Geometry check sheet. Reference: the model listing, model coordinates, mm. A direction names the side the tool comes from. Round coordinates to 2 decimals unless told otherwise and drop trailing zeros. Order: outer loops, then holes, each group sorted by start corner. A loop starts at its lowest first (then second) coordinate and runs counter-clockwise, first axis right, second up.
```python
from build123d import *

# Parameters (mm, degrees)
EXTRUDE_1_DEPTH     = 70
SKETCH_2_R          = 1.65
CUT_EXTRUDE_1_DEPTH = 25.69615506
FILLET_1_R          = 3
SKETCH_6_R          = 2.65
CUT_EXTRUDE_4_DEPTH = 31.641777725
EXTRUDE_2_DEPTH     = 3
CUT_EXTRUDE_5_DEPTH = 31.641777725


with BuildPart() as part:
    # 草图1 → 凸台-拉伸1 (new body)
    with BuildSketch(Plane(origin=(0, 0, 0), x_dir=(0, 0, -1), z_dir=(1, 0, 0))):
        Polygon((0, 0), (90, 0), (64.288495613, -30.641777725), (60.458273397, -27.427839676), (79.277465397, -5), (0, -5), align=None)
    extrude(amount=EXTRUDE_1_DEPTH)

    # 草图2 → 切除-拉伸1 (cut, through all)
    with BuildSketch(Plane(origin=(0, -41.102410837, -48.983945779), x_dir=(1, 0, 0), z_dir=(0, 0.64278761, 0.766044443))):
        with Locations((12.5, 27.850884872)):
            Circle(SKETCH_2_R)
        with Locations((57.5, 27.850884872)):
            Circle(SKETCH_2_R)
    extrude(amount=-CUT_EXTRUDE_1_DEPTH, mode=Mode.SUBTRACT)

    # 圆角1
    fillet_1_edges = [part.edges().sort_by_distance(p)[0] for p in [
        (35, 0, -90),
        (35, -5, -79.277465397),
    ]]
    fillet(fillet_1_edges, radius=FILLET_1_R)

    # 草图6 → 切除-拉伸4 (cut, through all)
    with BuildSketch(Plane(origin=(0, 0, 0), x_dir=(1, 0, 0), z_dir=(0, 1, 0))):
        with Locations((48.75, 5)):
            Circle(SKETCH_6_R)
    extrude(amount=-CUT_EXTRUDE_4_DEPTH, mode=Mode.SUBTRACT)

    # 草图7 → 凸台-拉伸2 (add)
    with BuildSketch(Plane.ZY):
        with BuildLine():
            Line((-60.458273397, -27.427839676), (-15, -5))
            Line((-15, -5), (0, -5))
            Line((0, -5), (0, 0))
            Line((0, 0), (-83.566479238, 0))
            ThreePointArc((-83.566479238, 0), (-86.2854026, -1.732145215), (-85.864612568, -4.928362829))
            Line((-85.864612568, -4.928362829), (-64.288495613, -30.641777725))
            Line((-64.288495613, -30.641777725), (-60.458273397, -27.427839676))
        make_face()
    extrude_2 = extrude(amount=EXTRUDE_2_DEPTH)

    # 镜向1: 凸台-拉伸2 across plane
    add(extrude_2.mirror(Plane.ZY.offset(-35)))

    # 草图8 → 切除-拉伸5 (cut, through all)
    with BuildSketch(Plane(origin=(0, 0, 0), x_dir=(1, 0, 0), z_dir=(0, 1, 0))):
        with BuildLine():
            Line((16.25, 10.15), (26.25, 10.15))
            ThreePointArc((26.25, 10.15), (28.9, 7.5), (26.25, 4.85))
            Line((26.25, 4.85), (16.25, 4.85))
            ThreePointArc((16.25, 4.85), (13.6, 7.5), (16.25, 10.15))
        make_face()
    extrude(amount=-CUT_EXTRUDE_5_DEPTH, mode=Mode.SUBTRACT)


solid = part.part
```
(1) Material ranges on line 1 (X direction, y = -19.5, z = -60.5); line 2 (Y direction, x = 25.5, z = -42); line 3 (Z direction, x = 48.75, y = -2.15), recorded low to high.
Returned:
line 1: x = -3 to 0, 70 to 73
line 2: y = -5 to 0
line 3: z = -86.44 to -7.65, -2.35 to 0
(2) Sectioned sample at B-B, the plane z = -17. Record the cut outline in (x, y).
Returned:
outline: (-3, -5.99) - (0, -5.99) - (0, -5) - (70, -5) - (70, -5.99) - (73, -5.99) - (73, 0) - (-3, 0) - close
(3) Set-up check for faces 1 (the flat face through (73, -8, -54)), 2 (the cylindrical face through (35.49, -6.689, -75.542)), 3 (the flat face through (21, -2, -10.15)): record each of +Z, -Z, +X, -X, +Y, -Y from which the full face is reachable in a straight line by a thin tool's end or side.
Returned:
face 1: +Z, -Z, +X, +Y, -Y
face 2: +Z
face 3: +Y, -Y
(4) Depth check by flat-ended pin: P1, Ø10, axis at x = 24.5, y = -18, coming from the +Z side; P2, Ø5, axis at x = 11.5, z = -60, coming from the -Y side; P3, Ø8.5, axis at x = 48.75, z = -5, coming from the -Y side. Enter the tip coordinate at first touch or a pass-through.
Returned:
P1: stops at z = -64.17
P2: stops at y = -29.14
P3: stops at y = -5
(5) Sectioned sample at A-A, the plane x = 48.75. Record the cut outline in (y, z).
Returned:
outline: (-30.64, -64.29) - (-4.93, -85.86) arc R3 ccw to (0, -83.57) - (0, -7.65) - (-5, -7.65) - (-5, -72.84) arc R3 cw to (-9.93, -75.14) - (-27.43, -60.46) - close; (-5, -2.35) - (0, -2.35) - (0, 0) - (-5, 0) - close
(6) Sectioned sample at D-D, the plane y = -28.5. Record the cut outline in (x, z), and give its area (3 significant figures).
Returned:
outline: (-3, -66.09) - (73, -66.09) - (73, -61.74) - (-3, -61.74) - close
area: 331 mm2
(7) Draft check along Z on faces 4 (the flat face through (34, -3, 0)), 5 (the flat face through (34, 0, -41)), 6 (the cylindrical face through (28.9, -2.5, -7.6)). Enter one of: released by +Z, released by -Z, zero draft, split by the parting line, or undercut.
Returned:
face 4: released by +Z
face 5: zero draft
face 6: undercut
(8) Sectioned sample at C-C, the plane y = -7. Record the cut outline in (x, z).
Returned:
outline: (-3, -84.13) - (73, -84.13) - (73, -19.05) - (70, -19.05) - (70, -75.67) - (0, -75.67) - (0, -19.05) - (-3, -19.05) - close
